Check sheet for the modelled part. Datum: model origin and axes. Units: mm. Give positions to 0.01 mm unless a question says otherwise; leave off trailing zeros. Order: outer loops, then holes, each group sorted by start corner. A loop starts at its lowest first (then second) coordinate and runs counter-clockwise, first axis right, second up. Notation, with made-up numbers: (84, 19.25) - (118, 19.25) arc R22 ccw to (118, 30.25) - close; hole circle Ø7 at (11.5, 52.5). An arc over 180 degrees is marked (long way). Answer in a Markdown table with one row per item.
from build123d import *

# Parameters (mm, degrees)
F0_W     = 76.2
F0_H     = 101.6
F1_DEPTH = 50.8
F2_W     = 69.7807297111
F2_H     = 44.052880723
F3_DEPTH = 159.766
F4_W     = 76.2
F4_H     = 50.8
F5_DEPTH = 5.588
F6_W     = 76.2
F6_H     = 50.8
F7_DEPTH = 5.842
F8_R     = 10.042531578
F9_DEPTH = 166.116


with BuildPart() as f1:
    # F0 (on Top) → F1 (new body)
    with BuildSketch(Plane.XY):
        Rectangle(F0_W, F0_H)
    extrude(amount=F1_DEPTH)

    # F2 (on face) → F3 (cut)
    with BuildSketch(Plane.XZ.offset(50.8)):
        with Locations((-0.0047236681, 25.0930653419)):
            Rectangle(F2_W, F2_H)
    extrude(amount=-F3_DEPTH, mode=Mode.SUBTRACT)

    # F4 (on face) → F5 (join)
    with BuildSketch(Plane.XZ.offset(50.8)):
        with Locations((0, 25.4)):
            Rectangle(F4_W, F4_H)
    extrude(amount=F5_DEPTH)

    # F6 (on face) → F7 (join)
    with BuildSketch(Plane(origin=(0, 50.8, 0), x_dir=(-1, 0, 0), z_dir=(0, 1, 0))):
        with Locations((0, 25.4)):
            Rectangle(F6_W, F6_H)
    extrude(amount=F7_DEPTH)

    # F8 (on face) → F9 (cut)
    with BuildSketch(Plane.XZ.offset(56.388)):
        with Locations((0, 24.429988116)):
            Circle(F8_R)
    extrude(amount=-F9_DEPTH, mode=Mode.SUBTRACT)


solid = f1.part
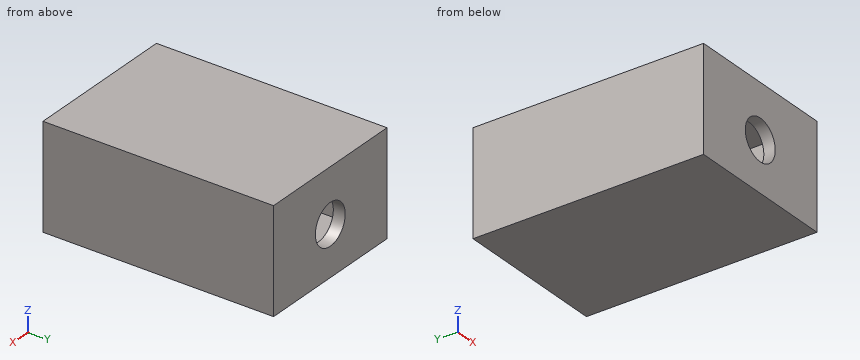
(1) Cross-section at B-B, the plane z = 17.5. Record the cut outline in (x, y).
Geometry says:
| item | result |
|---|---|
| outline | (-38.1, -56.39) - (-7.27, -56.39) - (-7.27, -50.8) - (-34.9, -50.8) - (-34.9, 50.8) - (-7.27, 50.8) - (-7.27, 56.64) - (-38.1, 56.64) - close; (7.27, -56.39) - (38.1, -56.39) - (38.1, 56.64) - (7.27, 56.64) - (7.27, 50.8) - (34.89, 50.8) - (34.89, -50.8) - (7.27, -50.8) - close |
(2) Cross-section at D-D, the plane z = 42. Record the cut outline in (x, y), then the cut area to 3 significant figures.
Geometry says:
| item | result |
|---|---|
| outline | (-38.1, -56.39) - (38.1, -56.39) - (38.1, 56.64) - (-38.1, 56.64) - close; hole (-34.9, -50.8) - (34.89, -50.8) - (34.89, 50.8) - (-34.9, 50.8) - close |
| area | 1,520 mm² |
(3) Cross-section at C-C, the plane y = 1. Record the cut outline in (x, z), then the cut area to 3 significant figures.
Geometry says:
| item | result |
|---|---|
| outline | (-38.1, 0) - (38.1, 0) - (38.1, 50.8) - (-38.1, 50.8) - close; hole (-34.9, 3.07) - (34.89, 3.07) - (34.89, 47.12) - (-34.9, 47.12) - close |
| area | 797 mm² |
(4) Thickness scan on L1, parallel to Z at x = 0, y = 53.1; L2, parallel to X at y = 26, z = 39; L3, parallel to Z at x = -17, y = 44. Record the ranges inside material, lowest first.
Geometry says:
| item | result |
|---|---|
| L1 | 0 to 14.39, 34.47 to 50.8 |
| L2 | -38.1 to -34.9, 34.89 to 38.1 |
| L3 | 0 to 3.07, 47.12 to 50.8 |
(5) Cross-section at A-A, the plane x = 0. Record the cut outline in (y, z).
Geometry says:
| item | result |
|---|---|
| outline | (-56.39, 0) - (56.64, 0) - (56.64, 14.39) - (50.8, 14.39) - (50.8, 3.07) - (-50.8, 3.07) - (-50.8, 14.39) - (-56.39, 14.39) - close; (-56.39, 34.47) - (-50.8, 34.47) - (-50.8, 47.12) - (50.8, 47.12) - (50.8, 34.47) - (56.64, 34.47) - (56.64, 50.8) - (-56.39, 50.8) - close |
